```python
from build123d import *

# Parameters (mm, degrees)
F0_W     = 101.6
F0_H     = 50.8000018598
F1_DEPTH = 25.4
F2_W     = 101.6
F2_H     = 50.8000018598
F2_W_2   = 3.8264841478
F2_H_2   = 32.9250585148
F3_DEPTH = 25.4


with BuildPart() as f1:
    # F0 (on Front) → F1 (new body)
    with BuildSketch(Plane.XZ):
        with Locations((-3.8295406848, 7.522309199)):
            Rectangle(F0_W, F0_H)
    extrude(amount=F1_DEPTH)

    # F2 (on face) → F3 (join)
    with BuildSketch(Plane.XZ.offset(25.4)):
        with Locations((-3.8295406848, 7.522309199)):
            Rectangle(F2_W, F2_H)
        Polygon((-30.1501307976, -1.3310039), (-30.1501307976, -4.797178806), (-52.7847573669, -4.797178806), (-52.7847573669, -1.7994059143), (-35.30975914, 24.6833233572), (-52.2442935042, 24.6833233572), (-52.2442935042, 28.1278797087), (-30.6473575513, 28.1278797087), (-30.6473575513, 25.1301068171), (-48.1223557781, -1.3310039), align=None, mode=Mode.SUBTRACT)
        Polygon((0.8797011054, -4.797178806), (-3.0837005543, -4.797178806), (-7.1840197259, 5.6734077604), (-20.3785441602, 5.6734077604), (-24.428420038, -4.797178806), (-28.3053474796, -4.797178806), (-15.2909776662, 28.2647972206), (-12.0698130446, 28.2647972206), align=None, mode=Mode.SUBTRACT)
        with Locations((7.3184272562, 11.6653504514)):
            Rectangle(F2_W_2, F2_H_2, mode=Mode.SUBTRACT)
        with BuildLine():
            Line((43.9798926083, 28.1278797087), (43.9798926083, -4.797178806))
            Line((43.9798926083, -4.797178806), (39.6129445978, -4.797178806))
            Line((39.6129445978, -4.797178806), (21.6191010628, 22.8313338544))
            Line((21.6191010628, 22.8313338544), (21.4389464419, 22.8313338544))
            add(Edge.make_bspline(
                [(21.4389464419, 22.8313338544), (21.7992556837, 17.9671590903), (21.7992556837, 13.9172832125)],
                knots=[0, 0, 0, 1, 1, 1], degree=2))
            Line((21.7992556837, 13.9172832125), (21.7992556837, -4.797178806))
            Line((21.7992556837, -4.797178806), (18.2610189293, -4.797178806))
            Line((18.2610189293, -4.797178806), (18.2610189293, 28.1278797087))
            Line((18.2610189293, 28.1278797087), (22.5847298308, 28.1278797087))
            Line((22.5847298308, 28.1278797087), (40.5353362568, 0.6074598208))
            Line((40.5353362568, 0.6074598208), (40.7154908777, 0.6074598208))
            add(Edge.make_bspline(
                [(40.7154908777, 0.6074598208), (40.6722537687, 1.212779347), (40.5137177023, 4.5132120018)],
                knots=[0, 0, 0, 1, 1, 1], degree=2))
            add(Edge.make_bspline(
                [(40.5137177023, 4.5132120018), (40.3551816359, 7.8136446566), (40.3984187449, 9.2332630693)],
                knots=[0, 0, 0, 1, 1, 1], degree=2))
            Line((40.3984187449, 9.2332630693), (40.3984187449, 28.1278797087))
            Line((40.3984187449, 28.1278797087), (43.9798926083, 28.1278797087))
        make_face(mode=Mode.SUBTRACT)
    extrude(amount=F3_DEPTH)


solid = f1.part
```
Geometry check sheet. Reference: the model listing, model coordinates, mm. A direction names the side the tool comes from. Coordinates: 2 decimals unless noted, no trailing zeros. Loops run counter-clockwise (first coordinate to the right, second up) from the corner with the lowest first, then second, coordinate; pieces in that order, holes last.
Item 1: Sectioned sample at B-B, the plane z = 12. Record the boundary of the cut face in (x, y).
Item 2: Sectioned sample at C-C, the plane y = -36. Count the separate pieces of the cut face and the enclosed holes in it, then the cut area to 3 significant figures.
Item 3: Sectioned sample at D-D, the plane z = 27. Record the boundary of the cut face in (x, y), then the cut area to 3 significant figures.
Item 4: Sectioned sample at A-A, the plane x = 6.5. Record the boundary of the cut face in (y, z).
Item 5: Thickness scan on line 1 (X direction, y = -26.5, z = 24); line 2 (Y direction, x = -8.5, z = 10). Record the ranges inside material, lowest first.
Item 6: Go/stop test with a flat-tipped pin: pin 1 Ø14.5 at (x, z) = (-12, 16.5) entering from -Y. Record where the tip stops, or that it passes through.
Item 7: Release check for a two-part mould opening along X. For faces 1 (the face through (46.97, -25, 7)), 2 (the face through (-5, -25, 32.922)), 3 (the face through (18.261, -38, 11)) record: released by +X, released by -X, zero draft, split by the parting line, or undercut.
Item 8: Access from +Z, -Z, +X, -X, +Y, -Y to the whole of each face (thin tool, end or side, straight path). Record for faces 4 (the face through (-5, 0, 8)), 5 (the face through (7, -25.4, 12)).
Check result:
1. outline: (-54.63, -50.8) - (-43.68, -50.8) - (-43.68, -25.4) - (-39.32, -25.4) - (-39.32, -50.8) - (-21.69, -50.8) - (-21.69, -25.4) - (-5.7, -25.4) - (-5.7, -50.8) - (5.41, -50.8) - (5.41, -25.4) - (9.23, -25.4) - (9.23, -50.8) - (18.26, -50.8) - (18.26, -25.4) - (21.8, -25.4) - (21.8, -50.8) - (28.67, -50.8) - (28.67, -25.4) - (33.1, -25.4) - (33.1, -50.8) - (40.4, -50.8) - (40.4, -25.4) - (43.98, -25.4) - (43.98, -50.8) - (46.97, -50.8) - (46.97, 0) - (-54.63, 0) - close
2. separate pieces: 1
2. enclosed holes: 4
2. area: 4,060 mm2
3. outline: (-54.63, -50.8) - (-52.24, -50.8) - (-52.24, -25.4) - (-30.65, -25.4) - (-30.65, -50.8) - (-15.79, -50.8) - (-15.79, -25.4) - (-11.57, -25.4) - (-11.57, -50.8) - (5.41, -50.8) - (5.41, -25.4) - (9.23, -25.4) - (9.23, -50.8) - (18.26, -50.8) - (18.26, -25.4) - (23.32, -25.4) - (23.32, -50.8) - (40.4, -50.8) - (40.4, -25.4) - (43.98, -25.4) - (43.98, -50.8) - (46.97, -50.8) - (46.97, 0) - (-54.63, 0) - close
3. area: 4,190 mm2
4. outline: (-50.8, -17.88) - (0, -17.88) - (0, 32.92) - (-50.8, 32.92) - (-50.8, 28.13) - (-25.4, 28.13) - (-25.4, -4.8) - (-50.8, -4.8) - close
5. line 1: x = -54.63 to -35.76, -31.39 to -16.97, -10.4 to 5.41, 9.23 to 18.26, 25.28 to 40.4, 43.98 to 46.97
5. line 2: y = -25.4 to 0
6. pin 1: stops at y = -50.8
7. face 1: released by +X
7. face 2: zero draft
7. face 3: undercut
8. face 4: +Z, -Z, +X, -X, +Y
8. face 5: -Y
